The listing builds one solid part. Answer for the finished solid, in the listing's coordinates (mm). Face numbers are marked on the shaded views. Coordinates: 2 decimals unless noted, no trailing zeros. Order: outer loops, then holes, each group sorted by start corner. A loop starts at its lowest first (then second) coordinate and runs counter-clockwise, first axis right, second up.
from build123d import *

# Parameters (mm, degrees)
BOSS_EXTRUDE1_DEPTH = 1185
SKETCH3_R           = 5
CUT_EXTRUDE1_DEPTH  = 20


with BuildPart() as part:
    # Sketch1 → Boss-Extrude1 (new body)
    with BuildSketch(Plane.XY):
        Polygon((3, -76.55), (76.2, -76.55), (76.2, -82.55), (-76.2, -82.55), (-76.2, -76.55), (-3, -76.55), (-3, 76.55), (-76.2, 76.55), (-76.2, 82.55), (76.2, 82.55), (76.2, 76.55), (3, 76.55), align=None)
    extrude(amount=BOSS_EXTRUDE1_DEPTH)

    # Sketch3 → Cut-Extrude1 (cut)
    with BuildSketch(Plane.XZ.offset(82.55)):
        with Locations(Location((-47.5, 1156.3, 0), (0, 0, 270))):
            Circle(SKETCH3_R)
        with Locations(Location((47.5, 1156.3, 0), (0, 0, 270))):
            Circle(SKETCH3_R)
        with Locations(Location((-47.5, 1016.3, 0), (0, 0, 270))):
            Circle(SKETCH3_R)
        with Locations(Location((47.5, 1016.3, 0), (0, 0, 270))):
            Circle(SKETCH3_R)
        with Locations(Location((47.5, 168.7, 0), (0, 0, 90))):
            Circle(SKETCH3_R)
        with Locations(Location((-47.5, 168.7, 0), (0, 0, 90))):
            Circle(SKETCH3_R)
        with Locations(Location((47.5, 28.7, 0), (0, 0, 90))):
            Circle(SKETCH3_R)
        with Locations(Location((-47.5, 28.7, 0), (0, 0, 90))):
            Circle(SKETCH3_R)
    extrude(amount=-CUT_EXTRUDE1_DEPTH, mode=Mode.SUBTRACT)


solid = part.part
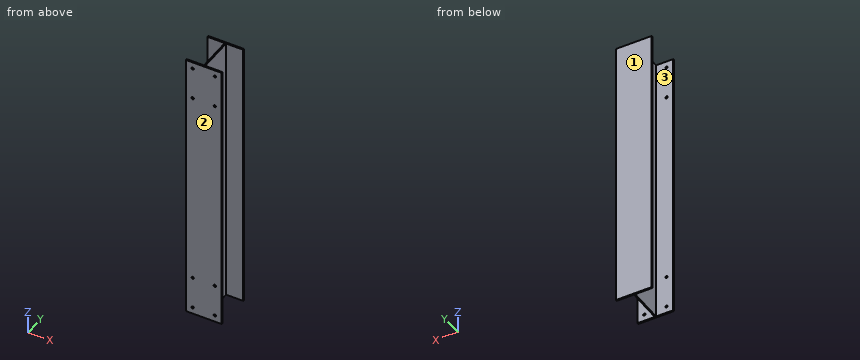
1) Section C-C (y = -7.5) is taken. Give the vertices of the cut face in (x, z).
2) Consider L1, parallel to X at y = -79, z = 28; L2, parallel to Y at x = -32.5, z = 356; L3, parallel to Z at x = 47, y = -78. Determine where each line is inside the solid, lowest interval first.
3) Section B-B (x = 15.5) is taken. Give the vertices of the cut face in (y, z), then the cut area to 3 significant figures.
4) Section A-A (z = 225.5) is taken. Give the vertices of the cut face in (x, y), then the cut area to 3 significant figures.
5) Determine the mould class of the marked faces 1, 2 and 3 for opening direction Y: released by +Y, released by -Y, zero draft, split by the parting line, or undercut.
6) Each of these flat-tipped pins is pushed along its axis until it touches: P1, Ø6, axis at x = 6.5, y = -49.5, coming from the +Z side; P2, Ø9, axis at x = -47.5, z = 1016.3, coming from the -Y side; P3, Ø3, axis at y = 18.5, z = 579.5, coming from the +X side. Where does it stop, or does it pass through?
Filled sheet:
1. outline: (-3, 0) - (3, 0) - (3, 1185) - (-3, 1185) - close
2. L1: x = -76.2 to -52.45, -42.55 to 42.55, 52.45 to 76.2
2. L2: y = -82.55 to -76.55, 76.55 to 82.55
2. L3: z = 0 to 23.73, 33.67 to 163.73, 173.67 to 1011.33, 1021.27 to 1151.33, 1161.27 to 1185
3. outline: (-82.55, 0) - (-76.55, 0) - (-76.55, 1185) - (-82.55, 1185) - close; (76.55, 0) - (82.55, 0) - (82.55, 1185) - (76.55, 1185) - close
3. area: 14,200 mm2
4. outline: (-76.2, -82.55) - (76.2, -82.55) - (76.2, -76.55) - (3, -76.55) - (3, 76.55) - (76.2, 76.55) - (76.2, 82.55) - (-76.2, 82.55) - (-76.2, 76.55) - (-3, 76.55) - (-3, -76.55) - (-76.2, -76.55) - close
4. area: 2,750 mm2
5. face 1: released by +Y
5. face 2: released by -Y
5. face 3: undercut
6. P1: passes through
6. P2: stops at y = 76.55
6. P3: stops at x = 3
